Design review of the part built by this model. Coordinates are the model's own, in mm. A direction names the side the tool comes from. Coordinates: 2 decimals unless noted, no trailing zeros. Write each loop counter-clockwise with the first axis right and the second up, starting at its lowest first coordinate (ties: lowest second). Pieces come first, ordered by that corner, then holes. Notation, with made-up numbers: M 22,66.25 L 77,66.25 A21 ccw 77,98.25 Z; hole C 80,65 d2. An arc over 180 degrees is marked long. Write item = value, one per line.
```python
from build123d import *

# Parameters (mm, degrees)
SKETCH1_W           = 150
SKETCH1_H           = 85
BOSS_EXTRUDE1_DEPTH = 2
SKETCH2_W           = 150
SKETCH2_H           = 85
SKETCH2_W_2         = 145
SKETCH2_H_2         = 80
BOSS_EXTRUDE2_DEPTH = 10
FILLET1_R           = 20
FILLET2_R           = 1


with BuildPart() as part:
    # Sketch1 → Boss-Extrude1 (new body)
    with BuildSketch(Plane(origin=(0, 0, 0), x_dir=(1, 0, 0), z_dir=(0, 1, 0))):
        Rectangle(SKETCH1_W, SKETCH1_H)
    extrude(amount=BOSS_EXTRUDE1_DEPTH)

    # Sketch2 → Boss-Extrude2 (add)
    with BuildSketch(Plane(origin=(0, 2, 0), x_dir=(1, 0, 0), z_dir=(0, 1, 0))):
        Rectangle(SKETCH2_W, SKETCH2_H)
        Rectangle(SKETCH2_W_2, SKETCH2_H_2, mode=Mode.SUBTRACT)
    extrude(amount=BOSS_EXTRUDE2_DEPTH)

    # Fillet1
    fillet1_edges = [part.edges().sort_by_distance(p)[0] for p in [
        (72.5, 7, -40),
        (-72.5, 7, -40),
        (-72.5, 7, 40),
        (72.5, 7, 40),
        (75, 6, 42.5),
        (-75, 6, 42.5),
        (-75, 6, -42.5),
        (75, 6, -42.5),
    ]]
    fillet(fillet1_edges, radius=FILLET1_R)

    # Fillet2
    fillet2_edges = [part.edges().sort_by_distance(p)[0] for p in [
        (0, 0, -42.5),
        (0, 12, -42.5),
        (75, 0, 0),
        (0, 0, 42.5),
        (-75, 0, 0),
        (-69.142135624, 0, -36.642135624),
        (-69.142135624, 0, 36.642135624),
        (69.142135624, 0, 36.642135624),
        (69.142135624, 0, -36.642135624),
        (75, 12, 0),
        (0, 12, 42.5),
        (-75, 12, 0),
        (-72.5, 12, 0),
        (0, 12, 40),
        (72.5, 12, 0),
        (0, 12, -40),
        (-66.642135624, 12, 34.142135624),
        (66.642135624, 12, 34.142135624),
        (66.642135624, 12, -34.142135624),
        (-66.642135624, 12, -34.142135624),
        (-69.142135624, 12, -36.642135624),
        (-69.142135624, 12, 36.642135624),
        (69.142135624, 12, 36.642135624),
        (69.142135624, 12, -36.642135624),
    ]]
    fillet(fillet2_edges, radius=FILLET2_R)


solid = part.part
```
Q1. Machinability: for faces 5 (the flat face through (-1, 6, 40)), 6 (the flat face through (-1, 6, 42.5)), which of the approach directions +Z, -Z, +X, -X, +Y, -Y give a long, thin tool a straight path to every point of the face, cutting with its end or side? Answer none if there is none.
Check result:
face_5 = +Y
face_6 = +Z, +X, -X, +Y, -Y
Q2. Wall thickness on line 1 (Z direction, x = 50, y = 8.75); line 2 (X direction, y = 9.5, z = -17); line 3 (Y direction, x = -30, z = -0.5): over which ranges is each line inside the solid? List them lowest first.
Check result:
line_1 = -42.5 to -40, 40 to 42.5
line_2 = -75 to -72.5, 72.5 to 75
line_3 = 0 to 2
Q3. For P1, Ø6, axis at x = -15.5, z = 5.5, coming from the +Y side; P2, Ø6, axis at y = 9, z = 30, coming from the +X side; P3, Ø6, axis at x = 59.5, y = 4, coming from the -Z side, all flat-tipped, find the tip position at first contact; note any pin that passes through.
Check result:
P1 = 2
P2 = 74.49
P3 = -42.44
Q4. Consider section B-B, the plane x = 46. State the section outline as (y, z) points, and give its area (3 significant figures).
Check result:
outline = M 0,-41.5 A1 ccw 1,-42.5 L 11,-42.5 A1 ccw 12,-41.5 L 12,-41 A1 ccw 11,-40 L 2,-40 L 2,40 L 11,40 A1 ccw 12,41 L 12,41.5 A1 ccw 11,42.5 L 1,42.5 A1 ccw 0,41.5 Z
area = 219 mm²
Q5. Consider section C-C, the plane z = 16. State the section outline as (x, y) points, and give its area (3 significant figures).
Check result:
outline = M -75,1 A1 ccw -74,0 L 74,0 A1 ccw 75,1 L 75,11 A1 ccw 74,12 L 73.5,12 A1 ccw 72.5,11 L 72.5,2 L -72.5,2 L -72.5,11 A1 ccw -73.5,12 L -74,12 A1 ccw -75,11 Z
area = 349 mm²
Q6. The part is to be moulded in two halves that separate along X. For faces 1 (the flat face through (-1, 0, -1)), 2 (the cylindrical face through (-66.797, 6.563, 33.986)), 3 (the cylindrical face through (-69.297, 6.07, 36.486)), 4 (the cylindrical face through (69.297, 5.93, -36.486)), say which applies: +X half, -X half, draft (parallel to the pull), parting line (faces both ways), or undercut.
Check result:
face_1 = draft
face_2 = undercut
face_3 = -X half
face_4 = +X half
Q7. Consider section A-A, the plane y = 8.75. State the section outline as (x, z) points.
Check result:
outline = M -75,-22.5 A20 ccw -55,-42.5 L 55,-42.5 A20 ccw 75,-22.5 L 75,22.5 A20 ccw 55,42.5 L -55,42.5 A20 ccw -75,22.5 Z; hole M -72.5,-20 A20 ccw -52.5,-40 L 52.5,-40 A20 ccw 72.5,-20 L 72.5,20 A20 ccw 52.5,40 L -52.5,40 A20 ccw -72.5,20 Z
